from build123d import *

# Parameters (mm, degrees)
F1_DEPTH = 1126
F2_R     = 6.75
F3_DEPTH = 6.190699014
F5_DEPTH = 34.7
F6_W     = 177.8
F6_H     = 101.9
F7_DEPTH = 6.4
F9_DEPTH = 6.4


with BuildPart() as f1:
    # F0 (on Front) → F1 (new body)
    with BuildSketch(Plane.XZ):
        Polygon((51, 50.95), (-51, 50.95), (-51, 45.3), (-2.825, 44.3), (-2.825, -44.3), (-51, -45.3), (-51, -50.95), (51, -50.95), (51, -45.3), (2.825, -44.3), (2.825, 44.3), (51, 45.3), align=None)
    extrude(amount=F1_DEPTH)

    # F2 (on face) → F3 (cut, through all)
    with BuildSketch(Plane(origin=(0, 0, -50.95), x_dir=(1, 0, 0), z_dir=(0, 0, -1))):
        with Locations((-31.75, 563)):
            Circle(F2_R)
        with Locations((31.75, 563)):
            Circle(F2_R)
        with Locations((-31.75, 486.8)):
            Circle(F2_R)
        with Locations((31.75, 486.8)):
            Circle(F2_R)
        with Locations((-31.75, 1018)):
            Circle(F2_R)
        with Locations((31.75, 1018)):
            Circle(F2_R)
        with Locations((-31.75, 941.8)):
            Circle(F2_R)
        with Locations((31.75, 941.8)):
            Circle(F2_R)
        with Locations((-31.75, 410.6)):
            Circle(F2_R)
        with Locations((31.75, 410.6)):
            Circle(F2_R)
        with BuildLine():
            Line((-27.5, 1046), (-27.5, 1113.3))
            ThreePointArc((-27.5, 1113.3), (-31.75, 1117.55), (-36, 1113.3))
            Line((-36, 1113.3), (-36, 1046))
            ThreePointArc((-36, 1046), (-31.75, 1041.75), (-27.5, 1046))
        make_face()
        with BuildLine():
            ThreePointArc((36, 1113.3), (31.75, 1117.55), (27.5, 1113.3))
            Line((27.5, 1113.3), (27.5, 1046))
            ThreePointArc((27.5, 1046), (31.75, 1041.75), (36, 1046))
            Line((36, 1046), (36, 1113.3))
        make_face()
        with Locations((-31.75, 201.2)):
            Circle(F2_R)
        with Locations((31.75, 201.2)):
            Circle(F2_R)
        with Locations((-31.75, 125)):
            Circle(F2_R)
        with Locations((31.75, 125)):
            Circle(F2_R)
    extrude(amount=-F3_DEPTH, mode=Mode.SUBTRACT)

    # F4 (on face) → F5 (join)
    with BuildSketch(Plane(origin=(0, 0, -50.95), x_dir=(1, 0, 0), z_dir=(0, 0, -1))):
        Polygon((51, 101.9), (-51, 101.9), (-51, 96.25), (-2.825, 95.25), (-2.825, 6.65), (-51, 5.65), (-51, 0), (51, 0), (51, 5.65), (2.825, 6.65), (2.825, 95.25), (51, 96.25), align=None)
    extrude(amount=F5_DEPTH)

    # F6 (on face) → F7 (join)
    with BuildSketch(Plane(origin=(0, 0, -85.65), x_dir=(1, 0, 0), z_dir=(0, 0, -1))):
        with Locations((0, 50.95)):
            Rectangle(F6_W, F6_H)
    extrude(amount=F7_DEPTH)

    # F8 (on face) → F9 (cut, through all)
    with BuildSketch(Plane(origin=(0, 0, -92.05), x_dir=(1, 0, 0), z_dir=(0, 0, -1))):
        with BuildLine():
            Line((-71.95, 17.3), (-71.95, 84.6))
            ThreePointArc((-71.95, 84.6), (-76.2, 88.85), (-80.45, 84.6))
            Line((-80.45, 84.6), (-80.45, 17.3))
            ThreePointArc((-80.45, 17.3), (-76.2, 13.05), (-71.95, 17.3))
        make_face()
        with BuildLine():
            ThreePointArc((80.45, 84.6), (76.2, 88.85), (71.95, 84.6))
            Line((71.95, 84.6), (71.95, 17.3))
            ThreePointArc((71.95, 17.3), (76.2, 13.05), (80.45, 17.3))
            Line((80.45, 17.3), (80.45, 84.6))
        make_face()
    extrude(amount=-F9_DEPTH, mode=Mode.SUBTRACT)


solid = f1.part
Build history of the part. All positions in model axes, mm. A direction names the side the tool comes from. Give positions to 0.01 mm unless a question says otherwise; leave off trailing zeros. Loops run counter-clockwise (first coordinate to the right, second up) from the corner with the lowest first, then second, coordinate; pieces in that order, holes last. Notation, with made-up numbers: (-7.5, 86.25) -> (18.5, 86.25) arc R27 ccw to (18.5, 103.25) -> close; hole circle Ø6 at (-20.75, 56). An arc over 180 degrees is marked (long way). Answer in a Markdown table with one row per item.
Item 1: Slice it at B-B on z = -73. Write the cut outline in (x, y) (3 decimals), plus the area to 3 significant figures.
Findings below:
| item | result |
|---|---|
| outline | (-51, -101.9) -> (51, -101.9) -> (51, -96.25) -> (2.825, -95.25) -> (2.825, -6.65) -> (51, -5.65) -> (51, 0) -> (-51, 0) -> (-51, -5.65) -> (-2.825, -6.65) -> (-2.825, -95.25) -> (-51, -96.25) -> close |
| area | 1,760 mm² |
Item 2: Slice it at D-D on x = 62. Write the cut outline in (y, z).
Findings below:
| item | result |
|---|---|
| outline | (-101.9, -92.05) -> (0, -92.05) -> (0, -85.65) -> (-101.9, -85.65) -> close |
Item 3: Slice it at C-C on y = -606. Write the cut outline in (x, z) (3 decimals).
Findings below:
| item | result |
|---|---|
| outline | (-51, -50.95) -> (51, -50.95) -> (51, -45.3) -> (2.825, -44.3) -> (2.825, 44.3) -> (51, 45.3) -> (51, 50.95) -> (-51, 50.95) -> (-51, 45.3) -> (-2.825, 44.3) -> (-2.825, -44.3) -> (-51, -45.3) -> close |
Item 4: Tool access for faces 5 (the flat face through (2.825, -555, -1)), 6 (the flat face through (51, -477, -50)), 7 (the flat face through (-2.825, -555, 1)), 8 (the flat face through (-46, -52, -85.65)), 9 (the flat face through (45, -52, -85.65)): list every direction of +Z, -Z, +X, -X, +Y, -Y with a clear straight run to the whole face (end or side of a thin tool).
Findings below:
| item | result |
|---|---|
| face 5 | +X, +Y, -Y |
| face 6 | +Z, +X, +Y, -Y |
| face 7 | -X, +Y, -Y |
| face 8 | -X |
| face 9 | +X |
Item 5: Probe line 1 along X through (y, z) = (-563, -48); line 2 along Z through (x, y) = (-42, -651.5); line 3 along Z through (x, y) = (-5.5, -648.5). List the from-to ranges inside material, lowest first. Write a range as [from, to].
Findings below:
| item | result |
|---|---|
| line 1 | x = [-51, -38.5], [-25, 25], [38.5, 51] |
| line 2 | z = [-50.95, -45.11], [45.11, 50.95] |
| line 3 | z = [-50.95, -44.36], [44.36, 50.95] |
Item 6: Mould opens along Y. For faces 1 (the flat face through (2.825, -50, -68)), 2 (the flat face through (-1, -101.9, -71)), 3 (the flat face through (-1, -607, -50.95)), 4 (the flat face through (27, -50, -50.95)) say: pulls with the +Y half, pulls with the -Y half, needs draft (parallel to the pull), parting line crosses it, or undercut.
Findings below:
| item | result |
|---|---|
| face 1 | undercut |
| face 2 | pulls with the -Y half |
| face 3 | needs draft |
| face 4 | undercut |
Item 7: Slice it at A-A on x = 13.5. Write the cut outline in (y, z), plus the area to 3 significant figures.
Findings below:
| item | result |
|---|---|
| outline | (-1126, -50.95) -> (-101.9, -50.95) -> (-101.9, -92.05) -> (0, -92.05) -> (0, -44.52) -> (-1126, -44.52) -> close; (-1126, 44.52) -> (0, 44.52) -> (0, 50.95) -> (-1126, 50.95) -> close; hole (-95.47, -85.65) -> (-6.43, -85.65) -> (-6.43, -50.95) -> (-95.47, -50.95) -> close |
| area | 15,600 mm² |
Item 8: Flat gauge pins, fed straight in: P1, Ø1.7, axis at y = -561, z = 49, coming from the +X side; P2, Ø6, axis at y = -493.5, z = 47.5, coming from the -X side; P3, Ø6, axis at x = 31.5, z = -60.5, coming from the -Y side; P4, Ø12, axis at x = 32.5, z = -55, coming from the -Y side. Where does each tip first touch, or does it go through?
Findings below:
| item | result |
|---|---|
| P1 | stops at x = 51 |
| P2 | stops at x = -51 |
| P3 | stops at y = -101.9 |
| P4 | stops at y = -1126 |
